Build history of the part. All positions in model axes, mm. Face numbers are marked on the shaded views. Give positions to 0.01 mm unless a question says otherwise; leave off trailing zeros. Return JSON: item names as keys, results as strings. Group by question number.
Q1. Flat gauge pins, fed straight in: pin 1 Ø6 at (y, z) = (3.5, -10) entering from +X; pin 2 Ø1 at (x, z) = (4, -70.5) entering from -Y; pin 3 Ø1 at (y, z) = (2, -72.5) entering from +X; pin 4 Ø4 at (x, y) = (5.5, 3) entering from -Z. Where does each tip first touch, or does it go through?
Q2. Wall check: probe 1 along Y at (x, z) = (-0.25, -50.5); probe 2 along Z at (x, y) = (1.5, -6); probe 3 along Y at (x, z) = (-1.5, -20.5). Give the ranges that are in metal, low to high.
Q3. Pull direction X, two halves, no side cores. Call the marked faces 1 and 2: +X half, -X half, draft (parallel to the pull), parting line (faces both ways), or undercut.
from build123d import *

# Parameters (mm, degrees)
SKETCH1_R           = 7.3025
BOSS_EXTRUDE1_DEPTH = 6.35
SKETCH2_R           = 4.445
BOSS_EXTRUDE2_DEPTH = 90.17


with BuildPart() as part:
    # Sketch1 → Boss-Extrude1 (new body)
    with BuildSketch(Plane.XY):
        Circle(SKETCH1_R)
    extrude(amount=BOSS_EXTRUDE1_DEPTH)

    # Sketch2 → Boss-Extrude2 (add)
    with BuildSketch(Plane.XY):
        Circle(SKETCH2_R)
    extrude(amount=-BOSS_EXTRUDE2_DEPTH)

    # Sketch8 → Revolve2 (revolve)
    with BuildSketch(Plane(origin=(0, 0, 0), x_dir=(0, 0, -1), z_dir=(1, 0, 0))):
        Polygon((10.053866594, 4.445), (13.868978205, 4.445), (12.376730728, 5.890229165), (11.54322298, 5.890229165), align=None)
        Polygon((86.357441717, 4.447477676), (86.35496404, 4.445), (90.17, 4.445), (88.677752523, 5.890229165), (87.844244775, 5.890229165), align=None)
        Polygon((84.032175557, 5.890229165), (82.539928081, 4.445), (86.35496404, 4.445), (86.352486364, 4.447477676), (84.865683306, 5.890229165), align=None)
        Polygon((78.727369797, 4.447477676), (78.724892121, 4.445), (82.539928081, 4.445), (81.047680604, 5.890229165), (80.214172856, 5.890229165), align=None)
        Polygon((76.402103638, 5.890229165), (74.909856162, 4.445), (78.724892121, 4.445), (78.722414445, 4.447477676), (77.235611386, 5.890229165), align=None)
        Polygon((71.097297878, 4.447477676), (71.094820202, 4.445), (74.909856162, 4.445), (73.417608685, 5.890229165), (72.584100937, 5.890229165), align=None)
        Polygon((68.772031719, 5.890229165), (67.279784243, 4.445), (71.094820202, 4.445), (71.092342526, 4.447477676), (69.605539467, 5.890229165), align=None)
        Polygon((64.954029018, 5.890229165), (63.464672632, 4.445), (67.279784243, 4.445), (65.787536766, 5.890229165), align=None)
        Polygon((61.141808498, 5.890229165), (59.649561022, 4.445), (63.464672632, 4.445), (61.975316246, 5.890229165), align=None)
        Polygon((55.837002738, 4.447477676), (55.834525062, 4.445), (59.649561022, 4.445), (58.157313545, 5.890229165), (57.323805797, 5.890229165), align=None)
        Polygon((53.511736579, 5.890229165), (52.019489102, 4.445), (55.834525062, 4.445), (55.832047386, 4.447477676), (54.345244327, 5.890229165), align=None)
        Polygon((49.693733878, 5.890229165), (48.204377492, 4.445), (52.019489102, 4.445), (50.527241626, 5.890229165), align=None)
        Polygon((45.881513358, 5.890229165), (44.389265881, 4.445), (48.204377492, 4.445), (46.715021106, 5.890229165), align=None)
        Polygon((40.576707598, 4.447477676), (40.574229922, 4.445), (44.389265881, 4.445), (42.897018405, 5.890229165), (42.063510657, 5.890229165), align=None)
        Polygon((38.251441439, 5.890229165), (36.759193962, 4.445), (40.574229922, 4.445), (40.571752246, 4.447477676), (39.084949187, 5.890229165), align=None)
        Polygon((32.946635679, 4.447477676), (32.944158003, 4.445), (36.759193962, 4.445), (35.266946486, 5.890229165), (34.433438737, 5.890229165), align=None)
        Polygon((30.62136952, 5.890229165), (29.129122043, 4.445), (32.944158003, 4.445), (32.941680327, 4.447477676), (31.454877268, 5.890229165), align=None)
        Polygon((25.31656376, 4.447477676), (25.314086083, 4.445), (29.129122043, 4.445), (27.636874566, 5.890229165), (26.803366818, 5.890229165), align=None)
        Polygon((22.991297601, 5.890229165), (21.499050124, 4.445), (25.314086083, 4.445), (25.311608407, 4.447477676), (23.824805349, 5.890229165), align=None)
        Polygon((17.68649184, 4.447477676), (17.684014164, 4.445), (21.499050124, 4.445), (20.006802647, 5.890229165), (19.173294899, 5.890229165), align=None)
        Polygon((15.361225681, 5.890229165), (13.868978205, 4.445), (17.684014164, 4.445), (17.681536488, 4.447477676), (16.19473343, 5.890229165), align=None)
    revolve(axis=Axis((0, 0, -90.17), (0, 0, -1)))


solid = part.part
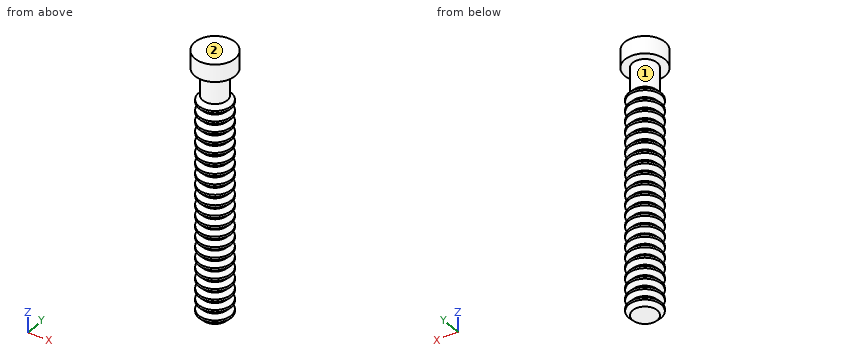
From the geometry:
{
 "1": {"pin 1": "stops at x = 5.82", "pin 2": "stops at y = -3.95", "pin 3": "stops at x = 5.69", "pin 4": "stops at z = -90.17"},
 "2": {"probe 1": "y = -5.88 to 5.88", "probe 2": "z = 0 to 6.35", "probe 3": "y = -5.2 to 5.2"},
 "3": {"face 1": "parting line", "face 2": "draft"}
}
